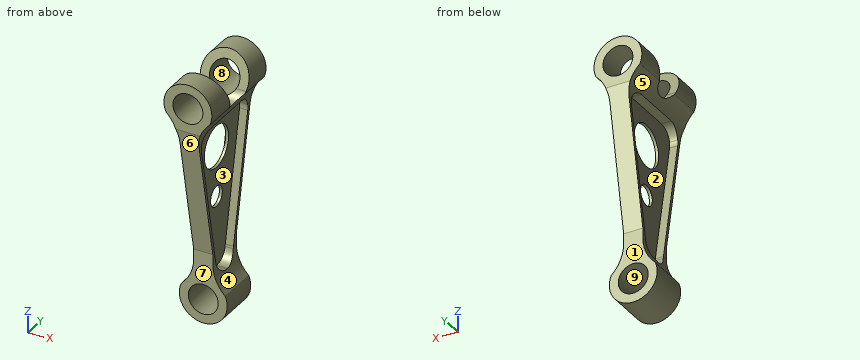
```python
from build123d import *

# Parameters (mm, degrees)
SKETCH2_R               = 19.84375
BOSS_EXTRUDE1_DEPTH     = 123.698
SKETCH3_R               = 19.05
CUT_EXTRUDE1_DEPTH      = 331.472839586
CUT_EXTRUDE1_DEPTH_BACK = 331.472839586
CUT_EXTRUDE2_START      = -10.795
CUT_EXTRUDE2_DEPTH      = 343.728785262


with BuildPart() as part:
    # Sketch2 → Boss-Extrude1 (new body)
    with BuildSketch(Plane(origin=(0, 0, 0), x_dir=(1, 0, 0), z_dir=(0, 1, 0))):
        with BuildLine():
            Line((-12.7, -50.079615691), (-12.7, -222.970384309))
            ThreePointArc((-12.7, -222.970384309), (-16.980150837, -243.379784933), (-29.099355663, -260.35))
            ThreePointArc((-29.099355663, -260.35), (0, -304.8), (29.099355663, -260.35))
            ThreePointArc((29.099355663, -260.35), (16.980150837, -243.379784933), (12.7, -222.970384309))
            Line((12.7, -222.970384309), (12.7, -50.079615691))
            ThreePointArc((12.7, -50.079615691), (16.980150837, -29.670215067), (29.099355663, -12.7))
            ThreePointArc((29.099355663, -12.7), (0, 31.75), (-29.099355663, -12.7))
            ThreePointArc((-29.099355663, -12.7), (-16.980150837, -29.670215067), (-12.7, -50.079615691))
        make_face()
        with Locations(Location((0, -273.05, 0), (0, 0, 270))):
            Circle(SKETCH2_R, mode=Mode.SUBTRACT)
        with Locations(Location((0, 0, 0), (0, 0, 270))):
            Circle(SKETCH2_R, mode=Mode.SUBTRACT)
    extrude(amount=BOSS_EXTRUDE1_DEPTH)

    # Sketch3 → Cut-Extrude1 (cut, two sides)
    with BuildSketch(Plane(origin=(0, 0, 0), x_dir=(0, 0, -1), z_dir=(1, 0, 0))) as cut_extrude1_sk:
        with BuildLine():
            Line((-289.037979654, 61.849), (-250.966020346, 61.849))
            ThreePointArc((-250.966020346, 61.849), (-270.002, 80.168261599), (-289.037979654, 61.849))
        make_face()
        with BuildLine():
            ThreePointArc((-289.037979654, 61.849), (-270.002, 43.529738401), (-250.966020346, 61.849))
            Line((-250.966020346, 61.849), (-289.037979654, 61.849))
        make_face()
        with Locations((-270.002, 61.118261599)):
            Circle(SKETCH3_R)
        with Locations((-270.002, 62.579738401)):
            Circle(SKETCH3_R)
        with BuildLine():
            ThreePointArc((-263.589413096, 43.18), (-281.270114367, 45.758180264), (-289.037979654, 61.849))
            Line((-289.037979654, 61.849), (-304.8, 61.849))
            Line((-304.8, 61.849), (-304.8, 28.448))
            Line((-304.8, 28.448), (-263.589413096, 43.18))
        make_face()
        with BuildLine():
            ThreePointArc((-289.037979654, 61.849), (-281.270114367, 77.939819736), (-263.589413096, 80.518))
            Line((-263.589413096, 80.518), (-304.8, 95.25))
            Line((-304.8, 95.25), (-304.8, 61.849))
            Line((-304.8, 61.849), (-289.037979654, 61.849))
        make_face()
        with BuildLine():
            ThreePointArc((-163.195, 61.849), (-191.008, 89.662), (-218.821, 61.849))
            Line((-218.821, 61.849), (-163.195, 61.849))
        make_face()
        with BuildLine():
            Line((-163.195, 61.849), (-218.821, 61.849))
            ThreePointArc((-218.821, 61.849), (-191.008, 34.036), (-163.195, 61.849))
        make_face()
        Polygon((31.75, 88.646), (-63.5, 88.646), (-241.3, 123.698), (31.75, 123.698), align=None)
        Polygon((31.75, 0), (31.75, 35.052), (-63.5, 35.052), (-241.3, 0), align=None)
        with BuildLine():
            ThreePointArc((-110.998, 61.849), (-124.46, 75.311), (-137.922, 61.849))
            Line((-137.922, 61.849), (-110.998, 61.849))
        make_face()
        with BuildLine():
            Line((-110.998, 61.849), (-137.922, 61.849))
            ThreePointArc((-137.922, 61.849), (-124.46, 48.387), (-110.998, 61.849))
        make_face()
    extrude(amount=CUT_EXTRUDE1_DEPTH, mode=Mode.SUBTRACT)
    extrude(cut_extrude1_sk.sketch, amount=-CUT_EXTRUDE1_DEPTH_BACK, mode=Mode.SUBTRACT)

    # Sketch4 → Cut-Extrude2 (cut)
    with BuildSketch(Plane(origin=(12.7, 0, 0), x_dir=(0, 0, -1), z_dir=(1, 0, 0)).offset(CUT_EXTRUDE2_START)):
        with BuildLine():
            Line((-50.079615691, 82.116934418), (-215.26334861, 114.681727479))
            ThreePointArc((-215.26334861, 114.681727479), (-219.120431461, 115.040686403), (-222.970384309, 114.611964231))
            Line((-222.970384309, 114.611964231), (-222.970384309, 61.849))
            Line((-222.970384309, 61.849), (-218.821, 61.849))
            ThreePointArc((-218.821, 61.849), (-191.008, 89.662), (-163.195, 61.849))
            Line((-163.195, 61.849), (-137.922, 61.849))
            ThreePointArc((-137.922, 61.849), (-124.46, 75.311), (-110.998, 61.849))
            Line((-110.998, 61.849), (-50.079615691, 61.849))
            Line((-50.079615691, 61.849), (-50.079615691, 82.116934418))
        make_face()
        with BuildLine():
            Line((-222.970384309, 61.849), (-222.970384309, 114.611964231))
            ThreePointArc((-222.970384309, 114.611964231), (-233.772454814, 107.955497873), (-237.998, 95.991466803))
            Line((-237.998, 95.991466803), (-237.998, 61.849))
            Line((-237.998, 61.849), (-222.970384309, 61.849))
        make_face()
        with BuildLine():
            Line((-222.970384309, 9.086035769), (-222.970384309, 61.849))
            Line((-222.970384309, 61.849), (-237.998, 61.849))
            Line((-237.998, 61.849), (-237.998, 27.706533197))
            ThreePointArc((-237.998, 27.706533197), (-233.772454814, 15.742502127), (-222.970384309, 9.086035769))
        make_face()
        with BuildLine():
            Line((-50.079615691, 41.581065582), (-50.079615691, 61.849))
            Line((-50.079615691, 61.849), (-110.998, 61.849))
            ThreePointArc((-110.998, 61.849), (-124.46, 48.387), (-137.922, 61.849))
            Line((-137.922, 61.849), (-163.195, 61.849))
            ThreePointArc((-163.195, 61.849), (-191.008, 34.036), (-218.821, 61.849))
            Line((-218.821, 61.849), (-222.970384309, 61.849))
            Line((-222.970384309, 61.849), (-222.970384309, 9.086035769))
            ThreePointArc((-222.970384309, 9.086035769), (-219.120431461, 8.657313597), (-215.26334861, 9.016272521))
            Line((-215.26334861, 9.016272521), (-50.079615691, 41.581065582))
        make_face()
        with BuildLine():
            Line((-31.75, 61.849), (-50.079615691, 61.849))
            Line((-50.079615691, 61.849), (-50.079615691, 41.581065582))
            Line((-50.079615691, 41.581065582), (-47.11534861, 42.165449664))
            ThreePointArc((-47.11534861, 42.165449664), (-36.084445152, 48.757985533), (-31.75, 60.85571034))
            Line((-31.75, 60.85571034), (-31.75, 61.849))
        make_face()
        with BuildLine():
            Line((-47.11534861, 81.532550336), (-50.079615691, 82.116934418))
            Line((-50.079615691, 82.116934418), (-50.079615691, 61.849))
            Line((-50.079615691, 61.849), (-31.75, 61.849))
            Line((-31.75, 61.849), (-31.75, 62.84228966))
            ThreePointArc((-31.75, 62.84228966), (-36.084445152, 74.940014467), (-47.11534861, 81.532550336))
        make_face()
    cut_extrude2 = extrude(amount=CUT_EXTRUDE2_DEPTH, mode=Mode.SUBTRACT)

    # Mirror1: Cut-Extrude2 across plane
    add(cut_extrude2.mirror(Plane(origin=(0, 0, 0), x_dir=(0, 0, 1), z_dir=(1, 0, 0))), mode=Mode.SUBTRACT)


solid = part.part
```
Design review of the part built by this model. Coordinates are the model's own, in mm. Face numbers are marked on the shaded views. A direction names the side the tool comes from. Round coordinates to 2 decimals unless told otherwise and drop trailing zeros. Write each loop counter-clockwise with the first axis right and the second up, starting at its lowest first coordinate (ties: lowest second). Pieces come first, ordered by that corner, then holes.
Item 1: We need section D-D on z = 115.5. Write out the cut boundary in (x, y) (3 decimals).
Item 2: The part is to be moulded in two halves that separate along Z. For the marked faces 6, 7, 8 and 9, say which applies: +Z half, -Z half, draft (parallel to the pull), parting line (faces both ways), or undercut.
Item 3: We need section C-C on x = -6.5. State how many separate pieces and enclosed holes the cut face has, and give its area (3 significant figures).
Item 4: We need section B-B on z = 273.05. Write out the cut boundary in (x, y).
Item 5: Clearance check with flat-ended pins moving along their axes: pin 1 Ø6 at (x, y) = (17, 52.5) entering from +Z; pin 2 Ø2 at (x, y) = (6, 62) entering from +Z; pin 3 Ø5 at (y, z) = (38.5, 217.5) entering from +X (3 decimals). State where each tip first meets the part, or that it passes through.
Item 6: For probe 1 along X at (y, z) = (73, 0); probe 2 along Z at (x, y) = (0, 76); probe 3 along Z at (x, y) = (9.5, 62.5), list the stretches that pass through material, from the lowest coordinate up.
Item 7: For the marked faces 1, 2, 3, 4 and 5, list the 3-axis set-ups (+Z, -Z, +X, -X, +Y, -Y) from which the entire face can be reached by the end or side of a thin tool; tool diameter is ignored.
Item 8: We need section A-A on z = 0. Write out the cut boundary in (x, y), and give its area (3 significant figures).
Returned:
1. outline: (-12.7, 24.801) - (12.7, 24.801) - (12.7, 28.684) - (1.905, 28.684) - (1.905, 51.802) - (-1.905, 51.802) - (-1.905, 28.684) - (-12.7, 28.684) - close; (-12.7, 95.014) - (-1.905, 95.014) - (-1.905, 71.896) - (1.905, 71.896) - (1.905, 95.014) - (12.7, 95.014) - (12.7, 98.897) - (-12.7, 98.897) - close
2. face 6: -Z half
2. face 7: draft
2. face 8: undercut
2. face 9: undercut
3. separate pieces: 4
3. enclosed holes: 1
3. area: 6,220 mm2
4. outline: (-31.75, 0) - (-19.84, 0) - (-19.84, 39.8) - (-31.75, 39.8) - close; (-31.75, 83.9) - (-19.84, 83.9) - (-19.84, 123.7) - (-31.75, 123.7) - close; (19.84, 0) - (31.75, 0) - (31.75, 39.8) - (19.84, 39.8) - close; (19.84, 83.9) - (31.75, 83.9) - (31.75, 123.7) - (19.84, 123.7) - close
5. pin 1: stops at z = 254.91
5. pin 2: stops at z = 250.97
5. pin 3: stops at x = 1.905
6. probe 1: x = -31.75 to -19.84, 19.84 to 31.75
6. probe 2: z = -31.75 to -19.84, 19.84 to 167.06, 214.95 to 253.21
6. probe 3: z = -30.3 to -17.42, 17.42 to 31.75, 238 to 250.95
7. face 1: -Z, +X, -X, +Y
7. face 2: -X
7. face 3: +X
7. face 4: +X, +Y, -Y
7. face 5: -X, +Y, -Y
8. outline: (-31.75, 35.05) - (-19.84, 35.05) - (-19.84, 88.65) - (-31.75, 88.65) - close; (19.84, 35.05) - (31.75, 35.05) - (31.75, 88.65) - (19.84, 88.65) - close
8. area: 1,280 mm2
